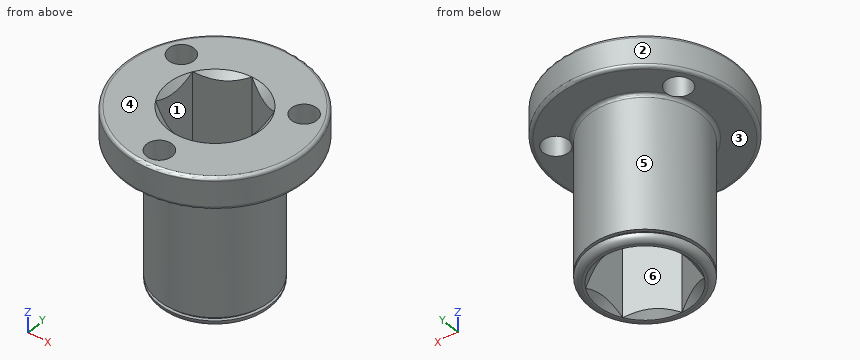
```python
from build123d import *

# Parameters (mm, degrees)
SKETCH2_R          = 3.96875
CUT_EXTRUDE1_DEPTH = 69.062067304


with BuildPart() as part:
    # Sketch1 → Revolve1 (revolve)
    with BuildSketch(Plane(origin=(0, 0, 0), x_dir=(0, 0, -1), z_dir=(1, 0, 0)), mode=Mode.PRIVATE) as revolve1_sk:
        with BuildLine():
            Line((0, 27.35), (0, 0))
            Line((0, 0), (55, 0))
            Line((55, 0), (55, 15.4625))
            ThreePointArc((55, 15.4625), (54.414213562, 16.876713562), (53, 17.4625))
            Line((53, 17.4625), (53, 16.5))
            Line((53, 16.5), (52, 16.5))
            Line((52, 16.5), (52, 17.4625))
            Line((52, 17.4625), (11, 17.4625))
            ThreePointArc((11, 17.4625), (10.292893219, 17.755393219), (10, 18.4625))
            Line((10, 18.4625), (10, 27.35))
            ThreePointArc((10, 27.35), (9.707106781, 28.057106781), (9, 28.35))
            Line((9, 28.35), (1, 28.35))
            ThreePointArc((1, 28.35), (0.292893219, 28.057106781), (0, 27.35))
        make_face()
    revolve(revolve1_sk.sketch.rotate(Axis((0, 0, 0), (0, 0, -1)), 90), axis=Axis((0, 0, 0), (0, 0, -1)))

    # Sketch2 → Cut-Extrude1 (cut, through all)
    with BuildSketch(Plane.XY):
        Polygon((0, 14.664696837), (-12.7, 7.332348419), (-12.7, -7.332348419), (0, -14.664696837), (12.7, -7.332348419), (12.7, 7.332348419), align=None)
        with Locations((-19.05, 10.998522628)):
            Circle(SKETCH2_R)
        with Locations((19.05, 10.998522628)):
            Circle(SKETCH2_R)
        with Locations((0, -21.997045256)):
            Circle(SKETCH2_R)
    extrude(amount=-CUT_EXTRUDE1_DEPTH, mode=Mode.SUBTRACT)

    # Sketch3 → Cut-Revolve2 (revolve, cut)
    with BuildSketch(Plane(origin=(0, 0, 0), x_dir=(0, 0, -1), z_dir=(1, 0, 0))):
        Polygon((0, 14.664696837), (0, 11.164696837), (3.5, 11.164696837), align=None)
        Polygon((51.5, 11.164696837), (55, 11.164696837), (55, 14.664696837), align=None)
    revolve(axis=Axis((0, 0, -55), (0, 0, 1)), mode=Mode.SUBTRACT)


solid = part.part
```
Can you work these out from the model? Positions are in its coordinate system, mm. Face numbers are marked on the shaded views. A direction names the side the tool comes from. Coordinates: 2 decimals unless noted, no trailing zeros. Loops run counter-clockwise (first coordinate to the right, second up) from the corner with the lowest first, then second, coordinate; pieces in that order, holes last.
1) Which directions (+Z, -Z, +X, -X, +Y, -Y) give clear straight access to the entire face, cutting with the end or side of a thin tool? Please do the marked faces 4, 5 and 6.
2) I need wall thicknesses on probe 1 along Y at (x, z) = (0, -4); probe 2 along Z at (x, y) = (-22.5, -9.5); probe 3 along Y at (x, z) = (-3, -14.5). Which ranges of each line are inside material? Lowest first, please.
3) For pin 1 (1.5 mm diameter, centred on x = 6.5, z = -10.5, fed in from -Y); pin 2 (8 mm diameter, centred on x = -16, z = -24, fed in from -Y); pin 3 (4.5 mm diameter, centred on y = -1, z = -35.5, fed in from -X); pin 4 (12.5 mm diameter, centred on x = 19.05, y = 11, fed in from +Z), each with a flat end and sliding along its axis, tell me the tip position at first contact or that it passes through.
4) Imagine slicing it at B-B on z = -50.5. List the corners of the cut face in (x, y) for me (1 decimal).
5) Thinking about a two-plate mould opening in Y: for the marked faces 1, 2 and 3, which applies, pulls with the +Y half, pulls with the -Y half, needs draft (parallel to the pull), parting line crosses it, or undercut?
6) Imagine slicing it at C-C on x = -2.5. State how many separate pieces and enclosed holes the cut face has, plus the area to 3 significant figures.
Completed:
1. face 4: +Z, +X, -X, +Y, -Y
1. face 5: -Z
1. face 6: +Z, -Z
2. probe 1: y = -28.35 to -25.97, -18.03 to -14.66, 14.66 to 28.35
2. probe 2: z = -10 to 0
2. probe 3: y = -17.2 to -12.93, 12.93 to 17.2
3. pin 1: stops at y = -27.26
3. pin 2: stops at y = -12.69
3. pin 3: stops at x = -17.46
3. pin 4: stops at z = 0
4. outline: circle Ø34.9 at (0, 0); hole (-12.7, -7.3) - (0, -14.7) - (12.7, -7.3) - (12.7, 7.3) - (0, 14.7) - (-12.7, 7.3) - close
5. face 1: undercut
5. face 2: parting line crosses it
5. face 3: needs draft
6. separate pieces: 3
6. enclosed holes: 0
6. area: 597 mm2
